Check sheet for the modelled part. Datum: model origin and axes. Units: mm. A direction names the side the tool comes from. Round coordinates to 2 decimals unless told otherwise and drop trailing zeros. Loops run counter-clockwise (first coordinate to the right, second up) from the corner with the lowest first, then second, coordinate; pieces in that order, holes last. Notation, with made-up numbers: (78, -11.75) - (113, -11.75) arc R29 ccw to (113, 9.25) - close; hole circle Ø1 at (-10.5, 87). An arc over 180 degrees is marked (long way). Answer in a Markdown table with one row per item. Add a question column.
(1) Thickness scan on line 1 along Y through (x, z) = (0.6, 6); line 2 along Y through (x, z) = (0.6, -11); line 3 along Z through (x, y) = (3.5, -4.5). Record the ranges inside material, lowest first.
(2) Gauge pin test, flat ends, axial feed: pin 1 (2.5 mm diameter, centred on x = 2, y = 54.5, fed in from -Z); pin 2 (3 mm diameter, centred on x = 1, y = 13, fed in from -Z). Record the tip position at first contact, or that the pin passes through.
(3) Cross-section at B-B on y = -5. Enter the section's corners in (x, z).
(4) Cross-section at C-C on x = 3. Enter the section's corners in (y, z).
(5) Cross-section at A-A on z = -5.5. Enter the section's corners in (x, y).
(6) Cross-section at D-D on y = 24.5. Enter the section's corners in (x, z).
(7) Access from +Z, -Z, +X, -X, +Y, -Y to the whole of each face (thin tool, end or side, straight path). Record for faces 5 (the flat face through (2, 48.534, 3)), 6 (the flat face through (2, 18, 15)), 7 (the flat face through (2, -31, 45)).
(8) Mould release check, pull along Y, two halves, no side actions. Record for faces 1 (the flat face through (2, 58.534, 7)), 2 (the flat face through (2, 53, -10)), 3 (the flat face through (2, 8.534, -10)), 4 (the cylindrical face through (3.475, -1.606, -8.314)): +Y half, -Y half, draft (parallel to the pull), parting line (faces both ways), or undercut.
Autodesk Inventor part; units mm, degrees
ref_plane "YZ Plane" through (0, 0, 0) normal (1, 0, 0) x (0, 1, 0)
ref_plane "XZ Plane" through (0, 0, 0) normal (0, 1, 0) x (-1, 0, 0)
ref_plane "XY Plane" through (0, 0, 0) normal (0, 0, 1) x (1, 0, 0)
sketch "Sketch1" plane through (0, 0, 0) normal (1, 0, 0) x (0, 1, 0)
  line L0 (-21.3033, 45) -> (-41.466, 45)
  line L1 (-41.466, 45) -> (-41.466, -15)
  line L2 (-41.466, -15) -> (-11.466, -15)
  line L3 (-11.466, -15) -> (-11.466, 15)
  line L4 (-11.466, 15) -> (48.534, 15)
  line L5 (48.534, 15) -> (48.534, -10)
  line L6 (48.534, -10) -> (58.534, -10)
  line L7 (58.534, -10) -> (58.534, 25.2188)
  line L8 (58.534, 25.2188) -> (9.0933, 33.9365)
  line L9 (9.0933, 33.9365) -> (-21.3033, 45)
  point P0 (0, 0)
  dimension "d0" = 60
  dimension "d1" = 30
  dimension "d2" = 30
  dimension "d3" = 60
  dimension "d4" = 10
  dimension "d5" = 100
  dimension "d7" = 25
  dimension "d8" = 160
  dimension "d9" = 58.534
  dimension "d10" = 10
  dimension "d11" = 35
  dimension "d12" = 35
extrude "Extrusion1" add sketch "Sketch1" along normal blind 5
sketch "Sketch2" plane through (0, -11.466, 15) normal (0, 1, 0) x (1, 0, 0)
  circle A0 centre (2.4001, 25) radius 2
  line L0 (0, 30) -> (0, 0)
  line L1 (0, 0) -> (5, 0)
  line L2 (5, 30) -> (5, 0)
  line L3 (0, 30) -> (5, 30)
  point P0 (0, 15)
  dimension "d15" = 4
  dimension "d16" = 25
extrude "Extrusion2" add sketch "Sketch2" along normal blind 20 contours A0
properties part number "Pala1"
Answers:
| question | item | result |
|---|---|---|
| 1 | line 1 | y = -41.47 to -11.47, 48.53 to 58.53 |
| 1 | line 2 | y = -41.47 to -11.47 |
| 1 | line 3 | z = -11.67 to -8.33, 15 to 38.88 |
| 2 | pin 1 | stops at z = -10 |
| 2 | pin 2 | stops at z = 15 |
| 3 | outline | (0, 15) - (5, 15) - (5, 39.07) - (0, 39.07) - close; circle Ø4 at (2.4, -10) |
| 4 | outline | (-41.47, -15) - (-11.47, -15) - (-11.47, -11.91) - (8.53, -11.91) - (8.53, -8.09) - (-11.47, -8.09) - (-11.47, 15) - (48.53, 15) - (48.53, -10) - (58.53, -10) - (58.53, 25.22) - (9.09, 33.94) - (-21.3, 45) - (-41.47, 45) - close |
| 5 | outline | (0, -41.47) - (5, -41.47) - (5, -11.47) - (0, -11.47) - close; (0, 48.53) - (5, 48.53) - (5, 58.53) - (0, 58.53) - close |
| 6 | outline | (0, 15) - (5, 15) - (5, 31.22) - (0, 31.22) - close |
| 7 | face 5 | -Z, +X, -X |
| 7 | face 6 | +X, -X |
| 7 | face 7 | +Z, +X, -X, +Y, -Y |
| 8 | face 1 | +Y half |
| 8 | face 2 | draft |
| 8 | face 3 | undercut |
| 8 | face 4 | undercut |
